Design review of the part built by this model. Coordinates are the model's own, in mm. A direction names the side the tool comes from. Round coordinates to 2 decimals unless told otherwise and drop trailing zeros. Write each loop counter-clockwise with the first axis right and the second up, starting at its lowest first coordinate (ties: lowest second). Pieces come first, ordered by that corner, then holes. Notation, with made-up numbers: M 7,17.5 L 55,17.5 A17 cw 55,29.5 Z; hole C 22.25,-3.75 d4. An arc over 180 degrees is marked long. Use CSV: the item, a comma, the result in double quotes.
from build123d import *

# Parameters (mm, degrees)
SKETCH_1_R          = 32.5
SKETCH_1_R_2        = 1.2
EXTRUDE_1_DEPTH     = 1.5
CUT_EXTRUDE_1_DEPTH = 46.986411036
CUT_EXTRUDE_2_DEPTH = 43.74049602
SKETCH_4_R          = 1.5
SKETCH_4_R_2        = 1
EXTRUDE_2_DEPTH     = 5
FILLET_1_R          = 1
CUT_EXTRUDE_3_DEPTH = 5


with BuildPart() as part:
    # 草图1 → 凸台-拉伸1 (new body)
    with BuildSketch(Plane(origin=(0, 0, 0), x_dir=(1, 0, 0), z_dir=(0, 1, 0))):
        with Locations(Location((0, 0, 0), (0, 0, 270))):
            Circle(SKETCH_1_R)
        with Locations(Location((21.213203436, 21.213203436, 0), (0, 0, 270))):
            Circle(SKETCH_1_R_2, mode=Mode.SUBTRACT)
        with Locations(Location((21.213203436, -21.213203436, 0), (0, 0, 270))):
            Circle(SKETCH_1_R_2, mode=Mode.SUBTRACT)
        with Locations(Location((-21.213203436, -21.213203436, 0), (0, 0, 270))):
            Circle(SKETCH_1_R_2, mode=Mode.SUBTRACT)
        with Locations(Location((-21.213203436, 21.213203436, 0), (0, 0, 270))):
            Circle(SKETCH_1_R_2, mode=Mode.SUBTRACT)
    extrude(amount=EXTRUDE_1_DEPTH)

    # 草图2 → 切除-拉伸1 (cut, through all)
    with BuildSketch(Plane(origin=(0, 1.5, 0), x_dir=(1, 0, 0), z_dir=(0, 1, 0))):
        with BuildLine():
            Line((30.203476621, 12), (27.203476621, 12))
            Line((27.203476621, 12), (27.203476621, -12))
            Line((27.203476621, -12), (30.203476621, -12))
            ThreePointArc((30.203476621, -12), (32.5, 0), (30.203476621, 12))
        make_face()
        with BuildLine():
            Line((12, -27.203476621), (-12, -27.203476621))
            Line((-12, -27.203476621), (-12, -30.203476621))
            ThreePointArc((-12, -30.203476621), (0, -32.5), (12, -30.203476621))
            Line((12, -30.203476621), (12, -27.203476621))
        make_face()
        with BuildLine():
            Line((-27.203476621, -12), (-27.203476621, 12))
            Line((-27.203476621, 12), (-30.203476621, 12))
            ThreePointArc((-30.203476621, 12), (-32.5, 0), (-30.203476621, -12))
            Line((-30.203476621, -12), (-27.203476621, -12))
        make_face()
        with BuildLine():
            Line((-12, 27.203476621), (12, 27.203476621))
            Line((12, 27.203476621), (12, 30.203476621))
            ThreePointArc((12, 30.203476621), (0, 32.5), (-12, 30.203476621))
            Line((-12, 30.203476621), (-12, 27.203476621))
        make_face()
    extrude(amount=-CUT_EXTRUDE_1_DEPTH, mode=Mode.SUBTRACT)

    # 草图3 → 切除-拉伸2 (cut, through all)
    with BuildSketch(Plane(origin=(0, 1.5, 0), x_dir=(1, 0, 0), z_dir=(0, 1, 0))):
        Polygon((17, 26.25), (-17, 26.25), (-27.149655647, 26.25), (-14.240374978, 46.745445694), (28.149411973, 26.25), align=None)
    extrude(amount=-CUT_EXTRUDE_2_DEPTH, mode=Mode.SUBTRACT)

    # 草图4 → 凸台-拉伸2 (add)
    with BuildSketch(Plane(origin=(0, 1.5, 0), x_dir=(1, 0, 0), z_dir=(0, 1, 0))):
        with Locations(Location((22.203476621, 3, 0), (0, 0, 270))):
            Circle(SKETCH_4_R)
        with Locations(Location((18.203476621, 3, 0), (0, 0, 270))):
            Circle(SKETCH_4_R)
        with Locations(Location((24.203476621, -6, 0), (0, 0, 270))):
            Circle(SKETCH_4_R_2)
        with Locations(Location((24.203476621, -3, 0), (0, 0, 270))):
            Circle(SKETCH_4_R_2)
        with Locations(Location((21.203476621, -6, 0), (0, 0, 270))):
            Circle(SKETCH_4_R_2)
        with Locations(Location((21.203476621, -3, 0), (0, 0, 270))):
            Circle(SKETCH_4_R_2)
    extrude(amount=EXTRUDE_2_DEPTH)

    # 圆角1
    fillet_1_edges = [part.edges().sort_by_distance(p)[0] for p in [
        (22.203476621, 6.5, -4.5),
        (18.203476621, 6.5, -4.5),
        (24.203476621, 6.5, 5),
        (24.203476621, 6.5, 2),
        (21.203476621, 6.5, 5),
        (21.203476621, 6.5, 2),
    ]]
    fillet(fillet_1_edges, radius=FILLET_1_R)

    # 草图5 → 切除-拉伸3 (cut)
    with BuildSketch(Plane(origin=(0, 1.5, 0), x_dir=(1, 0, 0), z_dir=(0, 1, 0))):
        Polygon((12, -30.203476621), (12, 30.744142548), (-38.712969595, 30.744142548), (-38.712969595, -27.203476621), align=None)
    extrude(amount=-CUT_EXTRUDE_3_DEPTH, mode=Mode.SUBTRACT)


with BuildPart() as body_2:
    # of the pieces the cut leaves, the one that is kept (cut_extrude_3_keep)
    add(part.part.solids().sort_by_distance((21.203476621, 5.5, 7))[0])


solid = body_2.part
1) Add section A-A on y = 0.75. Write out the cut boundary in (x, z), then the cut area to 3 significant figures.
Answers:
outline,"M 12,-26.25 L 19.16,-26.25 A32.5 ccw 30.2,-12 L 27.2,-12 L 27.2,12 L 30.2,12 A32.5 ccw 12,30.2 Z; hole C 21.21,-21.21 d2.4; hole C 21.21,21.21 d2.4"
area,"764 mm²"
2) Add section B-B on z = 3. Write out the cut boundary in (x, y).
Answers:
outline,"M 12,0 L 27.2,0 L 27.2,1.5 L 25.2,1.5 L 25.2,5.5 A1 ccw 23.2,5.5 L 23.2,1.5 L 22.2,1.5 L 22.2,5.5 A1 ccw 20.2,5.5 L 20.2,1.5 L 12,1.5 Z"
3) For pin 1 Ø1.2 at (x, y) = (29.5, 0.5) entering from -Z; pin 2 Ø1.9 at (x, z) = (21.21, -21.21) entering from +Y; pin 3 Ø1 at (x, y) = (18, 4.5) entering from +Z; pin 4 Ø0.8 at (y, z) = (1, 1) entering from +X, all flat-tipped, find the tip position at first contact; note any pin that passes through.
Answers:
pin 1,"z = -14.87"
pin 2,"through"
pin 3,"z = -1.5"
pin 4,"x = 27.2"
4) Machinability: for faces 4 (the face through (16, 1, -26.25)), 5 (the face through (27.203, 1, 0)), 6 (the face through (20.87, 3.47, -2.31)), which of the approach directions +Z, -Z, +X, -X, +Y, -Y give a long, thin tool a straight path to every point of the face, cutting with its end or side? Answer none if there is none.
Answers:
face 4,"-Z, +X, -X, +Y, -Y"
face 5,"+X, +Y, -Y"
face 6,"+Y"
5) Add section D-D on z = 19.5. Write out the cut boundary in (x, y).
Answers:
outline,"M 12,0 L 26,0 L 26,1.5 L 12,1.5 Z"
6) Wall thickness on line 1 along Y through (x, z) = (17.5, 18); line 2 along Z through (x, y) = (21.25, 0.5); line 3 along X through (y, z) = (2, -4): over which ranges is each line inside the solid? List them lowest first. Write a range as [from, to].
Answers:
line 1,"[0, 1.5]"
line 2,"[-24.59, -22.41], [-20.01, 20.01], [22.41, 24.59]"
line 3,"[17.09, 19.32], [21.09, 23.32]"
7) The part is to be moulded in two halves that separate along Z. For faces 1 (the face through (23.59, 3.47, 5.21)), 2 (the face through (16.87, 3.47, -2.31)), 3 (the face through (22.85, 0.74, 23.11)), say which applies: released by +Z, released by -Z, zero draft, split by the parting line, or undercut.
Answers:
face 1,"undercut"
face 2,"split by the parting line"
face 3,"released by +Z"
8) Add section C-C on y = 4.5. Write out the cut boundary in (x, z), then the cut area to 3 significant figures.
Answers:
outline,"C 18.2,-3 d3; C 21.2,3 d2; C 21.2,6 d2; C 22.2,-3 d3; C 24.2,3 d2; C 24.2,6 d2"
area,"26.7 mm²"
